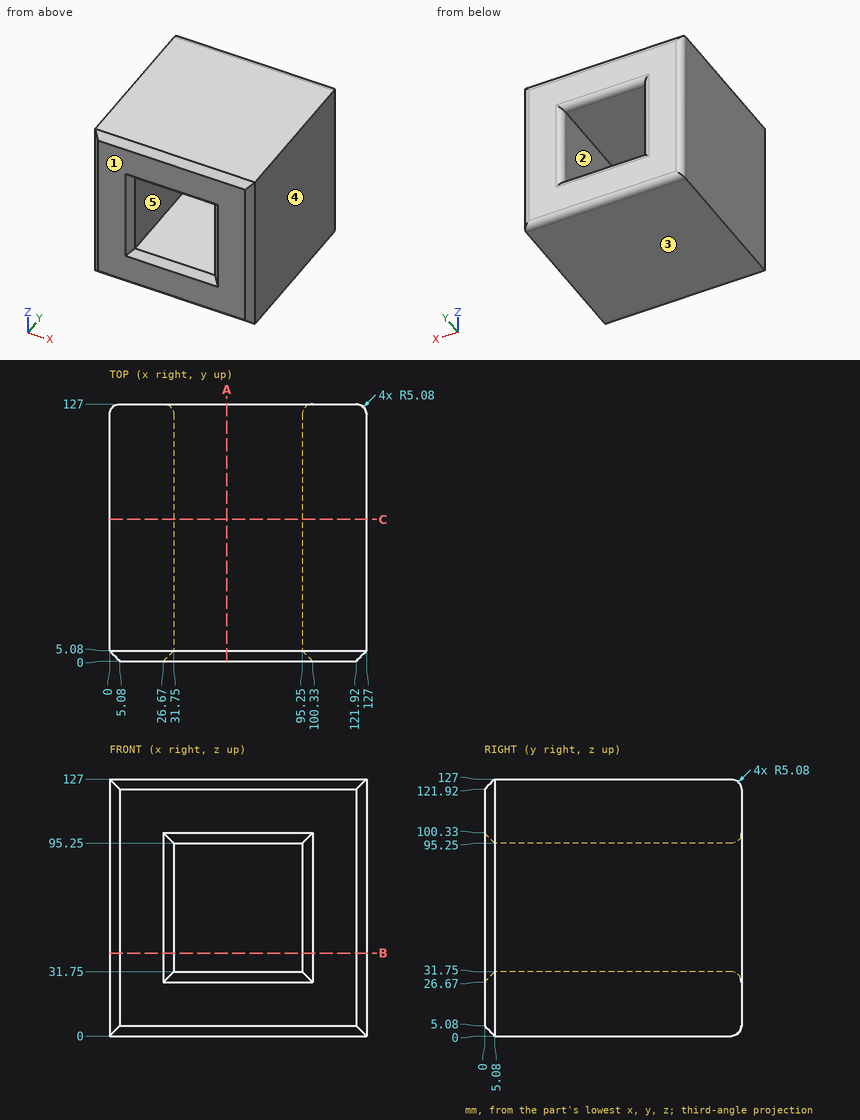
Verification items for this drawing (mm, ordinates from the low corner). A direction names the side the tool comes from. Give positions to 0.01 mm unless a question says otherwise; leave off trailing zeros. Loops run counter-clockwise (first coordinate to the right, second up) from the corner with the lowest first, then second, coordinate; pieces in that order, holes last. Notation, with made-up numbers: M -20.5,69.5 L 28.5,69.5 A19 cw 28.5,85.5 Z; hole C -24,32 d8. An arc over 180 degrees is marked long. Answer as a JSON object with one key per item and string values. Group by question number.
Q1. Access from +Z, -Z, +X, -X, +Y, -Y to the whole of each face (thin tool, end or side, straight path). Record for the marked faces 4 and 5.
Q2. Cross-section at C-C on y = 70. Record the cut outline in (x, z), then the cut area to 3 significant figures.
Q3. Cross-section at A-A on x = 58. Record the cut outline in (y, z), then the cut area to 3 significant figures.
Q4. Release check for a two-part mould opening along Z. For the marked faces 1, 2 and 3 record: released by +Z, released by -Z, zero draft, split by the parting line, or undercut.
Q5. Cross-section at B-B on z = 41. Record the cut outline in (x, y), then the cut area to 3 significant figures.
Q6. Material ranges on line 1 along X through (y, z) = (78.5, 58.5); line 2 along Y through (x, z) = (98, 47), recorded low to high. Write a range as [from, to].
Evaluation:
{
 "1": {"face 4": "+Z, -Z, +X, +Y, -Y", "face 5": "+Y, -Y"},
 "2": {"outline": "M 0,0 L 127,0 L 127,127 L 0,127 Z; hole M 31.75,31.75 L 95.25,31.75 L 95.25,95.25 L 31.75,95.25 Z", "area": "12,100 mm2"},
 "3": {"outline": "M 0,5.08 L 5.08,0 L 121.92,0 A5.08 ccw 127,5.08 L 127,26.67 A5.08 ccw 121.92,31.75 L 5.08,31.75 L 0,26.67 Z; M 0,100.33 L 5.08,95.25 L 121.92,95.25 A5.08 ccw 127,100.33 L 127,121.92 A5.08 ccw 121.92,127 L 5.08,127 L 0,121.92 Z", "area": "7,990 mm2"},
 "4": {"face 1": "zero draft", "face 2": "undercut", "face 3": "released by -Z"},
 "5": {"outline": "M 0,5.08 L 5.08,0 L 26.67,0 L 31.75,5.08 L 31.75,121.92 A5.08 ccw 26.67,127 L 5.08,127 A5.08 ccw 0,121.92 Z; M 95.25,5.08 L 100.33,0 L 121.92,0 L 127,5.08 L 127,121.92 A5.08 ccw 121.92,127 L 100.33,127 A5.08 ccw 95.25,121.92 Z", "area": "7,990 mm2"},
 "6": {"line 1": "x = [0, 31.75], [95.25, 127]", "line 2": "y = [2.33, 126.43]"}
}
